Could you check a few things on this model? Use its own coordinates, in mm. Face numbers are marked on the shaded views. A direction names the side the tool comes from. Give positions to 0.01 mm unless a question says otherwise; leave off trailing zeros. Order: outer loops, then holes, each group sorted by start corner. A loop starts at its lowest first (then second) coordinate and runs counter-clockwise, first axis right, second up. Notation, with made-up numbers: M 18.25,5 L 50.25,5 A22 ccw 50.25,16 Z; hole C -3,-5 d10. An arc over 180 degrees is marked long. Use a Markdown table: item, result. Add a question column.
Item 1: Suppose I cut it at A-A on x = 9. Write out the boundary of the cut face in (y, z), plus the area to 3 significant figures.
Item 2: I'm going to push flat-ended pins straight in: pin 1 Ø0.6 at (x, z) = (1.5, 1.5) entering from +Y; pin 2 Ø1 at (x, z) = (-16.5, 1.5) entering from -Y; pin 3 Ø2 at (y, z) = (7.5, 1.5) entering from +X. Where does each tip first touch, or does it pass through?
Item 3: Suppose I cut it at C-C on z = 4.5. Write out the boundary of the cut face in (x, y).
Item 4: If I drill on L1, parallel to Y at x = -22, z = 3.4; L2, parallel to Z at x = -12, y = -6; L3, parallel to Z at x = 8, y = -2.5, over which ranges is the centre line in solid material (lowest first)? Write a range as from..to.
Item 5: If we mould it in two halves opening along Y, with no side actions, what happens to the marked faces 1, 2 and 3? For each: released by +Y, released by -Y, zero draft, split by the parting line, or undercut.
Item 6: Suppose I cut it at B-B on x = -6.5. Write out the boundary of the cut face in (y, z).
Item 7: Suppose I cut it at D-D on x = -22. Write out the boundary of the cut face in (y, z).
Item 8: For the marked faces 4 and 5, which set-ups out of +Z, -Z, +X, -X, +Y, -Y let a thin tool reach every point of the face, with its end or its side?
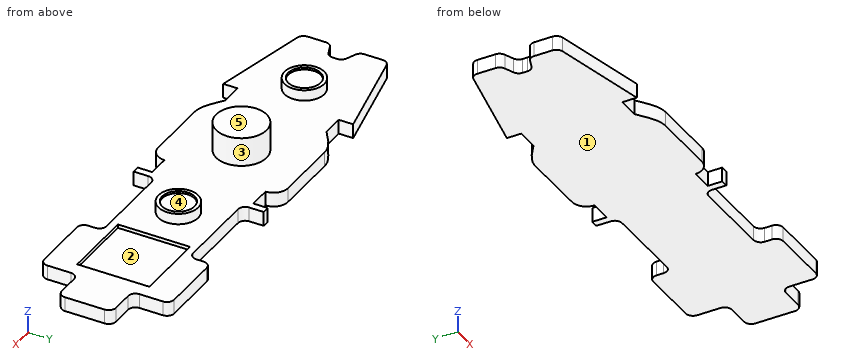
from build123d import *

# Parameters (mm, degrees)
F1_DEPTH  = 2
F2_R      = 1
F4_DEPTH  = 0.5
F5_R      = 2.75
F6_DEPTH  = 1.5
F7_R      = 2.25
F8_DEPTH  = 0.3
F9_R      = 3.5
F10_DEPTH = 2.5


with BuildPart() as f1:
    # F0 (on Top) → F1 (new body)
    with BuildSketch(Plane.XY):
        with BuildLine():
            Line((27, 4.75), (27, 9))
            Line((27, 9), (17, 9))
            Line((17, 9), (17, 7))
            ThreePointArc((17, 7), (16.707107, 6.292893), (16, 6))
            Line((16, 6), (5, 6))
            ThreePointArc((5, 6), (4.292893, 6.292893), (4, 7))
            Line((4, 7), (4, 9))
            Line((4, 9), (3, 9))
            Line((3, 9), (3, 7))
            Line((3, 7), (0, 7))
            ThreePointArc((0, 7), (-0.585786, 8.414214), (-2, 9))
            Line((-2, 9), (-11, 9))
            add(Edge.make_bspline(
                [(-15, 7), (-13.666667, 8), (-12.333333, 9), (-11, 9)],
                knots=[0, 0, 0, 0, 4.472136, 4.472136, 4.472136, 4.472136], degree=3))
            Line((-15, 7), (-18, 7))
            Line((-18, 7), (-18, 9))
            Line((-18, 9), (-32, 6))
            Line((-32, 6), (-32, 2))
            Line((-32, 2), (-30.128609, 1.251444))
            ThreePointArc((-30.128609, 1.251444), (-29.671933, 0.883596), (-29.5, 0.322967))
            Line((-29.5, 0.322967), (-29.5, 0))
            Line((-29.5, 0), (-29.5, -0.322967))
            ThreePointArc((-29.5, -0.322967), (-29.671933, -0.883596), (-30.128609, -1.251444))
            Line((-30.128609, -1.251444), (-31.371391, -1.748556))
            ThreePointArc((-31.371391, -1.748556), (-31.828067, -2.116404), (-32, -2.677033))
            Line((-32, -2.677033), (-32, -5.191584))
            ThreePointArc((-32, -5.191584), (-31.777666, -5.820262), (-31.209529, -6.169387))
            Line((-31.209529, -6.169387), (-18, -9))
            Line((-18, -9), (-18, -7))
            Line((-18, -7), (-15, -7))
            add(Edge.make_bspline(
                [(-15, -7), (-13.666667, -8), (-12.333333, -9), (-11, -9)],
                knots=[0, 0, 0, 0, 4.472136, 4.472136, 4.472136, 4.472136], degree=3))
            Line((-11, -9), (-2, -9))
            ThreePointArc((-2, -9), (-0.585786, -8.414214), (0, -7))
            Line((0, -7), (3, -7))
            Line((3, -7), (3, -9))
            Line((3, -9), (4, -9))
            Line((4, -9), (4, -7))
            ThreePointArc((4, -7), (4.292893, -6.292893), (5, -6))
            Line((5, -6), (16, -6))
            ThreePointArc((16, -6), (16.707107, -6.292893), (17, -7))
            Line((17, -7), (17, -8))
            ThreePointArc((17, -8), (17.292893, -8.707107), (18, -9))
            Line((18, -9), (26, -9))
            ThreePointArc((26, -9), (26.707107, -8.707107), (27, -8))
            Line((27, -8), (27, -4.75))
            ThreePointArc((27, -4.75), (27.292893, -4.042893), (28, -3.75))
            Line((28, -3.75), (32, -3.75))
            Line((32, -3.75), (32, 0))
            Line((32, 0), (32, 3.75))
            Line((32, 3.75), (28, 3.75))
            ThreePointArc((28, 3.75), (27.292893, 4.042893), (27, 4.75))
        make_face()
    extrude(amount=F1_DEPTH)

    # F2
    f2_edges = [f1.edges().sort_by_distance(p)[0] for p in [
        (-32, 2, 1),
        (-32, 6, 1),
        (27, 9, 1),
        (17, 9, 1),
        (32, -3.75, 1),
        (32, 3.75, 1),
    ]]
    fillet(f2_edges, radius=F2_R)

    # F3 (on face) → F4 (cut)
    with BuildSketch(Plane.XY.offset(2)):
        Polygon((25, -5), (25, 0), (25, 5), (15, 5), (15, -5), align=None)
    extrude(amount=-F4_DEPTH, mode=Mode.SUBTRACT)

    # F5 (on face) → F6 (join)
    with BuildSketch(Plane.XY.offset(2)):
        with BuildLine():
            ThreePointArc((6.25, 0), (9, -2.75), (11.75, 0))
            ThreePointArc((11.75, 0), (9, 2.75), (6.25, 0))
        make_face()
        with Locations((-22, 0)):
            Circle(F5_R)
        with BuildLine():
            ThreePointArc((-10, 0), (-6.5, -3.5), (-3, 0))
            ThreePointArc((-3, 0), (-6.5, 3.5), (-10, 0))
        make_face()
    extrude(amount=F6_DEPTH)

    # F7 (on face) → F8 (cut)
    with BuildSketch(Plane.XY.offset(3.5)):
        with Locations((9, 0)):
            Circle(F7_R)
        with Locations((-22, 0)):
            Circle(F7_R)
    extrude(amount=-F8_DEPTH, mode=Mode.SUBTRACT)

    # F9 (on face) → F10 (join)
    with BuildSketch(Plane.XY.offset(3.5)):
        with Locations((-6.5, 0)):
            Circle(F9_R)
    extrude(amount=F10_DEPTH)


solid = f1.part
Findings below:
| question | item | result |
|---|---|---|
| 1 | outline | M -6,0 L 6,0 L 6,2 L 2.75,2 L 2.75,3.5 L 2.25,3.5 L 2.25,3.2 L -2.25,3.2 L -2.25,3.5 L -2.75,3.5 L -2.75,2 L -6,2 Z |
| 1 | area | 30.9 mm^2 |
| 2 | pin 1 | stops at y = 7 |
| 2 | pin 2 | stops at y = -7 |
| 2 | pin 3 | stops at x = 27 |
| 3 | outline | C -6.5,0 d7 |
| 4 | L1 | y = -2.75..-2.25, 2.25..2.75 |
| 4 | L2 | z = 0..2 |
| 4 | L3 | z = 0..3.5 |
| 5 | face 1 | zero draft |
| 5 | face 2 | undercut |
| 5 | face 3 | split by the parting line |
| 6 | outline | M -9,0 L 9,0 L 9,2 L 3.5,2 L 3.5,6 L -3.5,6 L -3.5,2 L -9,2 Z |
| 7 | outline | M -8.14,0 L 8.14,0 L 8.14,2 L 2.75,2 L 2.75,3.5 L 2.25,3.5 L 2.25,3.2 L -2.25,3.2 L -2.25,3.5 L -2.75,3.5 L -2.75,2 L -8.14,2 Z |
| 8 | face 4 | +Z |
| 8 | face 5 | +Z, +X, -X, +Y, -Y |
